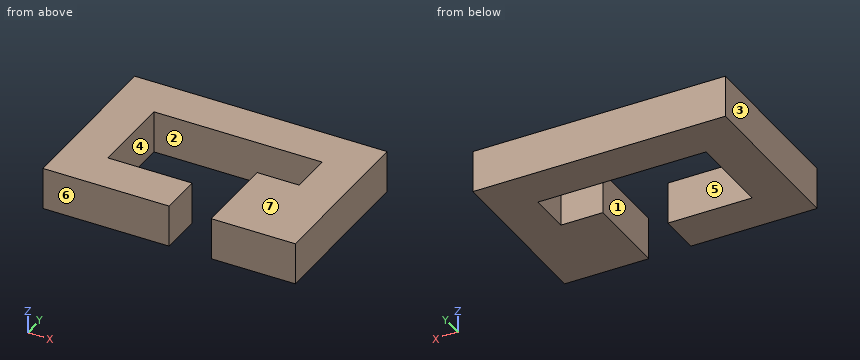
```python
from build123d import *

# Parameters (mm, degrees)
F0_W     = 10
F0_H     = 10
F1_DEPTH = 10


with BuildPart() as f1:
    # F0 (on Top) → F1 (new body)
    with BuildSketch(Plane.XY):
        Polygon((30, 20), (-30, 20), (-30, -20), (0, -20), (0, -10), (-20, -10), (-20, 10), (20, 10), (20, 0), (20, -10), (10, -10), (10, -20), (30, -20), align=None)
        with Locations((15, -5)):
            Rectangle(F0_W, F0_H)
    extrude(amount=F1_DEPTH)


solid = f1.part
```
The listing builds one solid part. Answer for the finished solid, in the listing's coordinates (mm). Face numbers are marked on the shaded views. A direction names the side the tool comes from. Give positions to 0.01 mm unless a question says otherwise; leave off trailing zeros. Order: outer loops, then holes, each group sorted by start corner. A loop starts at its lowest first (then second) coordinate and runs counter-clockwise, first axis right, second up. Notation, with made-up numbers: (-17, 21.25) -> (-4, 21.25) arc R15 cw to (-4, 39.25) -> close; hole circle Ø11 at (-18, -36). An arc over 180 degrees is marked (long way). Answer as a JSON object with one key per item and string values. Group by question number.
Item 1: Consider L1, parallel to Y at x = -14.5, z = 4.5; L2, parallel to X at y = 1, z = 3; L3, parallel to Y at x = 14, z = 9. Determine where each line is inside the solid, lowest interval first. Write a range as from..to.
Item 2: The part is cut by section B-B on x = -15. Write down the section's boundary in (y, z), and give its area (3 significant figures).
Item 3: The part is cut by section C-C on z = 1.25. Write down the section's boundary in (x, y), and give its area (3 significant figures).
Item 4: Determine the mould class of the marked faces 4, 5, 6 and 7 for opening direction Y: pulls with the +Y half, pulls with the -Y half, needs draft (parallel to the pull), parting line crosses it, or undercut.
Item 5: The part is cut by section D-D on x = 3.5. Write down the section's boundary in (y, z), and give its area (3 significant figures).
Item 6: A flat-ended cylindrical pin translates along its axis: pin 1 (12 mm diameter, centred on x = 0.5, y = -8.5, fed in from +Z). Find the tip coordinate at first contact, or state that the pin passes through.
Item 7: A tool of negligible diameter and unlimited length cuts with its end or side. For the marked faces 1, 2 and 3, from which of +Z, -Z, +X, -X, +Y, -Y can it reach the whole face along a straight path? Write none if from no direction.
Item 8: The part is cut by section A-A on y = -9. Write down the section's boundary in (x, z).
Result set:
{
 "1": {"L1": "-20..-10, 10..20", "L2": "-30..-20, 20..30", "L3": "-20..0, 10..20"},
 "2": {"outline": "(-20, 0) -> (-10, 0) -> (-10, 10) -> (-20, 10) -> close; (10, 0) -> (20, 0) -> (20, 10) -> (10, 10) -> close", "area": "200 mm²"},
 "3": {"outline": "(-30, -20) -> (0, -20) -> (0, -10) -> (-20, -10) -> (-20, 10) -> (20, 10) -> (20, 0) -> (10, 0) -> (10, -20) -> (30, -20) -> (30, 20) -> (-30, 20) -> close", "area": "1,600 mm²"},
 "4": {"face 4": "undercut", "face 5": "undercut", "face 6": "pulls with the -Y half", "face 7": "needs draft"},
 "5": {"outline": "(10, 0) -> (20, 0) -> (20, 10) -> (10, 10) -> close", "area": "100 mm²"},
 "6": {"pin 1": "z = 10"},
 "7": {"face 1": "+Z, -Z, -Y", "face 2": "+Z, -Z", "face 3": "+Z, -Z, -X, +Y, -Y"},
 "8": {"outline": "(-30, 0) -> (-20, 0) -> (-20, 10) -> (-30, 10) -> close; (10, 0) -> (30, 0) -> (30, 10) -> (10, 10) -> close"}
}
